Read the model definition and answer for the solid it produces. Units are mm, in the model's axes. Face numbers are marked on the shaded views. Give positions to 0.01 mm unless a question says otherwise; leave off trailing zeros. Loops run counter-clockwise (first coordinate to the right, second up) from the corner with the lowest first, then second, coordinate; pieces in that order, holes last. Notation, with made-up numbers: (-21.75, 25.25) - (31.25, 25.25) arc R21 cw to (31.25, 56.25) - close; hole circle Ø3 at (88, 47.5). An arc over 180 degrees is marked (long way). Use a Markdown table: item, result. Add a question column.
Item 1: A cutting plane is placed at A-A (y = -22). Determine the outline of the cut face in (x, z), plus the area to 3 significant figures.
Item 2: A cutting plane is placed at B-B (z = -19). Determine the outline of the cut face in (x, y), plus the area to 3 significant figures.
Item 3: Consider probe 1 along X at (y, z) = (-52, 0); probe 2 along X at (y, z) = (-42, 0); probe 3 along Z at (x, y) = (90, -44). Determine where each line is inside the solid, lowest interval first. Write a range as [from, to].
Item 4: For a pull along X with two mould halves and no side action, classify the marked faces 1, 2 and 3 as +X half, -X half, draft (parallel to the pull), parting line (faces both ways), or undercut.
Item 5: Each of these flat-tipped pins is pushed along its axis until it touches: P1, Ø20.5, axis at x = 60, z = 0, coming from the -Y side; P2, Ø12, axis at x = 68.5, y = -64, coming from the -Z side; P3, Ø2.5, axis at x = 58.5, z = -1, coming from the -Y side; P4, Ø6, axis at y = -65.5, z = 13.5, coming from the -X side. Where does it stop, or does it pass through?
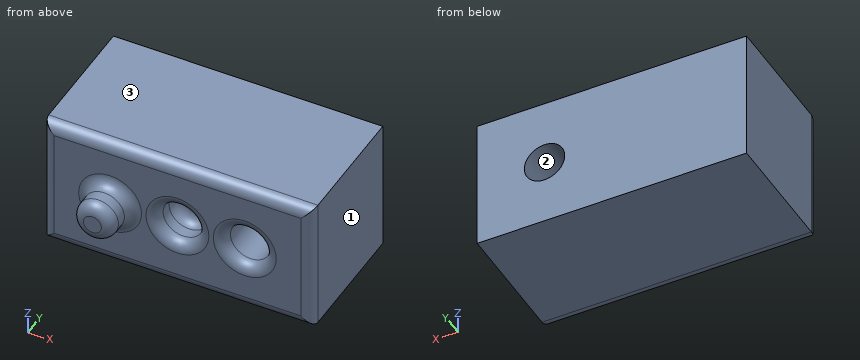
from build123d import *

# Parameters (mm, degrees)
F1_DEPTH = 60
F3_DEPTH = 75
F4_DEPTH = 45
F5_R     = 5
F6_R     = 5
F7_R     = 5


with BuildPart() as f1:
    # F0 (on Front) → F1 (new body)
    with BuildSketch(Plane.XZ):
        with BuildLine():
            ThreePointArc((81, 0), (90, 9), (99, 0))
            Line((99, 0), (120, 0))
            Line((120, 0), (120, 30))
            Line((120, 30), (0, 30))
            Line((0, 30), (0, 0))
            Line((0, 0), (21, 0))
            ThreePointArc((21, 0), (30, 9), (39, 0))
            Line((39, 0), (51, 0))
            ThreePointArc((51, 0), (60, 9), (69, 0))
            Line((69, 0), (81, 0))
        make_face()
        with BuildLine():
            Line((120, 0), (99, 0))
            ThreePointArc((99, 0), (90, -9), (81, 0))
            Line((81, 0), (69, 0))
            ThreePointArc((69, 0), (60, -9), (51, 0))
            Line((51, 0), (39, 0))
            ThreePointArc((39, 0), (30, -9), (21, 0))
            Line((21, 0), (0, 0))
            Line((0, 0), (0, -30))
            Line((0, -30), (120, -30))
            Line((120, -30), (120, 0))
        make_face()
    extrude(amount=F1_DEPTH)

    # F2 (on Front) → F3 (join)
    with BuildSketch(Plane.XZ):
        with BuildLine():
            ThreePointArc((39, 0), (30, 9), (21, 0))
            Line((21, 0), (30, 0))
            Line((30, 0), (39, 0))
        make_face()
        with BuildLine():
            Line((30, 0), (21, 0))
            ThreePointArc((21, 0), (30, -9), (39, 0))
            Line((39, 0), (30, 0))
        make_face()
    extrude(amount=F3_DEPTH)

    # F2 (on Front) → F4 (join)
    with BuildSketch(Plane.XZ):
        with BuildLine():
            ThreePointArc((69, 0), (60, 9), (51, 0))
            Line((51, 0), (60, 0))
            Line((60, 0), (69, 0))
        make_face()
        with BuildLine():
            Line((60, 0), (51, 0))
            ThreePointArc((51, 0), (60, -9), (69, 0))
            Line((69, 0), (60, 0))
        make_face()
    extrude(amount=F4_DEPTH)

    # F5
    f5_edges = [f1.edges().sort_by_distance(p)[0] for p in [
        (81, -60, 0),
        (60, -60, 30),
        (0, -60, 0),
        (60, -60, -30),
        (120, -60, 0),
        (39, -60, 0),
        (51, -60, 0),
    ]]
    fillet(f5_edges, radius=F5_R)

    # F6
    f6_edges = [f1.edges().sort_by_distance(p)[0] for p in [
        (39, -75, 0),
    ]]
    fillet(f6_edges, radius=F6_R)

    # F7
    f7_edges = [f1.edges().sort_by_distance(p)[0] for p in [
        (51, -45, 0),
    ]]
    fillet(f7_edges, radius=F7_R)


solid = f1.part
Geometry says:
| question | item | result |
|---|---|---|
| 1 | outline | (0, -30) - (120, -30) - (120, 30) - (0, 30) - close; hole circle Ø18 at (90, 0) |
| 1 | area | 6,950 mm² |
| 2 | outline | (0, -55) arc R5 ccw to (5, -60) - (115, -60) arc R5 ccw to (120, -55) - (120, 0) - (0, 0) - close |
| 2 | area | 7,190 mm² |
| 3 | probe 1 | [0, 51], [69, 81], [99, 120] |
| 3 | probe 2 | [0, 81], [99, 120] |
| 3 | probe 3 | [-30, -9], [9, 30] |
| 4 | face 1 | +X half |
| 4 | face 2 | undercut |
| 4 | face 3 | draft |
| 5 | P1 | y = -58.31 |
| 5 | P2 | z = -29 |
| 5 | P3 | y = -45 |
| 5 | P4 | through |
